Autodesk Inventor part; units mm, degrees
ref_plane "YZ Plane" through (0, 0, 0) normal (1, 0, 0) x (0, 1, 0)
ref_plane "XZ Plane" through (0, 0, 0) normal (0, 1, 0) x (-1, 0, 0)
ref_plane "XY Plane" through (0, 0, 0) normal (0, 0, 1) x (1, 0, 0)
sketch "Sketch1" plane through (0, 0, 0) normal (0, 1, 0) x (-1, 0, 0)
  line L0 (-13.25, -16.375) -> (13.25, -16.375)
  line L1 (13.25, -16.375) -> (13.25, 16.375)
  line L2 (13.25, 16.375) -> (-13.25, 16.375)
  line L3 (-13.25, 16.375) -> (-13.25, -16.375)
  line L4 (-13.25, -16.375) -> (13.25, 16.375) construction
  line L5 (13.25, -16.375) -> (-13.25, 16.375) construction
  point P0 (0, 0)
  dimension "d0" = 26.5
  dimension "d1" = 32.75
extrude "Extrusion1" add sketch "Sketch1" along normal blind 3.5 and the other way blind 11.5
shell "Shell1" thickness 1 removed faces 1 at (4.4167, -11.5, 5.4583)
sketch "Sketch2" plane through (0, 3.5, 0) normal (0, 1, 0) x (1, 0, 0)
  line L0 (13.25, 16.375) -> (-13.25, 16.375)
  line L1 (-13.25, 16.375) -> (-13.25, -16.375)
  line L2 (-13.25, -16.375) -> (13.25, -16.375)
  line L3 (13.25, -16.375) -> (13.25, 16.375)
  point P0 (0, 0)
extrude "Extrusion2" add sketch "Sketch2" along normal blind 1
sketch "Sketch3" plane through (-12.25, 2.5, -15.375) normal (0, -1, 0) x (1, 0, 0)
  line L0 (24.5, 0) -> (0, 0)
  line L1 (24.5, 30.75) -> (24.5, 0)
  line L2 (0, 30.75) -> (24.5, 30.75)
  line L3 (0, 0) -> (0, 30.75)
  line L4 (0.5, 3.625) -> (24, 3.625)
  line L5 (24, 3.625) -> (24, 27.125)
  line L6 (24, 27.125) -> (0.5, 27.125)
  line L7 (0.5, 27.125) -> (0.5, 3.625)
  circle A0 centre (12.25, 15.375) radius 11.75
  dimension "d9" = 0.5
  dimension "d10" = 0.5
  dimension "d11" = 3.625
  dimension "d12" = 3.625
  dimension "d13" = 23.5
  dimension "d14" = 23.5
extrude "Extrusion3" cut sketch "Sketch3" against normal blind 1 contours L7 A0 L4 | A0 L5 L4 | A0 | L7 L6 A0 | A0 L6 L5
extrude "Extrusion4" cut sketch "Sketch3" against normal blind 2 contours A0
sketch "Sketch4" plane through (-12.25, -11.5, -15.375) normal (0, 0, 1) x (1, 0, 0)
  line L0 (24.5, 0) -> (0, 0)
  line L1 (8.75, 6.5) -> (15.75, 6.5)
  line L2 (15.75, 6.5) -> (15.75, 0)
  line L3 (15.75, 0) -> (8.75, 0)
  line L4 (8.75, 0) -> (8.75, 6.5)
  line L5 (8.75, 6.5) -> (15.75, 0) construction
  line L6 (15.75, 6.5) -> (8.75, 0) construction
  circle A0 centre (12.25, 3.25) radius 3.5
  line L7 (15.75, 3.25) -> (15.75, 3.25)
  line L8 (8.75, 3.25) -> (8.75, 3.25)
  point P0 (12.25, 11.5)
  point P1 (12.25, 3.25)
  point P2 (12.25, 0)
  point P3 (12.25, 0)
  point P4 (10.951, 0)
  point P5 (13.549, 0)
  point P6 (15.75, 0)
  point P7 (15.75, 3.25)
  point P8 (8.75, 3.25)
  point P9 (8.75, 0)
  dimension "d19" = 7
  dimension "d20" = 6.5
  dimension "d21" = 7
  dimension "d22" = 3.25
  dimension "d23" = 3.25
extrude "Extrusion5" cut sketch "Sketch4" against normal blind 2 contours L0 A0 L2 | A0 L0 | L0 A0 L1 | L0 L4 A0 | L1 A0
sketch "Sketch5" plane through (-13.25, -11.5, -16.375) normal (-1, 0, 0) x (0, 0, 1)
  line L0 (0, 16) -> (32.75, 16)
  line L1 (30, 11) -> (3.2984, 11)
  line L2 (7, 11) -> (7, 3)
  line L3 (1, 0) -> (1, 14)
  line L4 (7, 4) -> (14, 4)
  line L5 (14, 4) -> (14, 11)
  line L6 (15.5, 11) -> (22.5, 11)
  line L7 (22.5, 11) -> (22.5, 4)
  line L8 (22.5, 4) -> (15.5, 4)
  line L9 (15.5, 4) -> (15.5, 11)
  point P0 (16.375, 11.5)
  dimension "d26" = 5
  dimension "d27" = 6
  dimension "d28" = 7
  dimension "d29" = 7
  dimension "d30" = 7
  dimension "d31" = 7
  dimension "d32" = 1.5
extrude "Extrusion6" cut sketch "Sketch5" against normal blind 2
sketch "Sketch6" plane through (0, -11.5, 0) normal (0, -1, 0) x (1, 0, 0)
  line L0 (3.5, -16.375) -> (13.25, -16.375)
  line L1 (13.25, -16.375) -> (13.25, 16.375)
  line L2 (13.25, 16.375) -> (-13.25, 16.375)
  line L3 (-13.25, 16.375) -> (-13.25, -16.375)
  line L4 (-13.25, -16.375) -> (-3.5, -16.375)
  line L5 (13.25, 16.375) -> (-13.25, 16.375)
  line L6 (-13.25, 16.375) -> (-13.25, -16.375)
  line L7 (-13.25, -16.375) -> (13.25, -16.375)
  line L8 (13.25, -16.375) -> (13.25, 16.375)
  point P0 (0, 0)
extrude "Extrusion7" add sketch "Sketch6" along normal blind 1
properties part number "carcasaXeotype_COLOR"
Part model, mm, in its own coordinate system. A direction names the side the tool comes from. Give positions to 0.01 mm unless a question says otherwise; leave off trailing zeros. Write each loop counter-clockwise with the first axis right and the second up, starting at its lowest first coordinate (ties: lowest second). Pieces come first, ordered by that corner, then holes.
1) Cut at B-B on x = -3. Write the cut outline in (y, z) (3 decimals), then the cut area to 3 significant figures.
Resolved:
outline: (-12.5, -16.375) - (-11.5, -16.375) - (-11.5, 15.375) - (2.5, 15.375) - (2.5, 11.75) - (3.5, 11.75) - (3.5, 11.361) - (4.5, 11.361) - (4.5, 16.375) - (-12.5, 16.375) - close; (-6.447, -16.375) - (4.5, -16.375) - (4.5, -11.361) - (3.5, -11.361) - (3.5, -11.75) - (2.5, -11.75) - (2.5, -15.375) - (-6.447, -15.375) - close
area: 75.0 mm2
2) Two-plate mould, pull along Z, no slides. Class faces 4 (the face through (-3.5, -10, -16)), 5 (the face through (0, -4, 16.375)), 6 (the face through (0, 3, -11.75)): released by +Z, released by -Z, zero draft, split by the parting line, or undercut.
Resolved:
face 4: zero draft
face 5: released by +Z
face 6: undercut
3) Cut at C-C on z = -10. Write the cut outline in (x, y).
Resolved:
outline: (-13.25, -12.5) - (13.25, -12.5) - (13.25, 4.5) - (6.17, 4.5) - (6.17, 3.5) - (11.75, 3.5) - (11.75, 2.5) - (12.25, 2.5) - (12.25, -11.5) - (-12.25, -11.5) - (-12.25, 2.5) - (-11.75, 2.5) - (-11.75, 3.5) - (-6.17, 3.5) - (-6.17, 4.5) - (-13.25, 4.5) - close
4) Cut at A-A on y = -1.75. Write the cut outline in (x, z) (3 decimals), then the cut area to 4 significant figures.
Resolved:
outline: (-13.25, -16.375) - (13.25, -16.375) - (13.25, 16.375) - (-13.25, 16.375) - (-13.25, 6.125) - (-12.25, 6.125) - (-12.25, 15.375) - (12.25, 15.375) - (12.25, -15.375) - (-12.25, -15.375) - (-12.25, -9.375) - (-13.25, -9.375) - close; (-13.25, -2.375) - (-12.25, -2.375) - (-12.25, -0.875) - (-13.25, -0.875) - close
area: 100.5 mm2
5) Cut at D-D on y = -9.75. Write the cut outline in (x, z) (3 decimals), then the cut area to 4 significant figures.
Resolved:
outline: (-13.25, -16.375) - (-3.5, -16.375) - (-3.5, -15.375) - (-12.25, -15.375) - (-12.25, 15.375) - (12.25, 15.375) - (12.25, -15.375) - (3.5, -15.375) - (3.5, -16.375) - (13.25, -16.375) - (13.25, 16.375) - (-13.25, 16.375) - close
area: 107.5 mm2
6) Probe L1, parallel to X at y = 4.25, z = 0; L2, parallel to X at y = -3.75, z = -14; L3, parallel to Z at x = -0.25, y = -0.25 (3 decimals). List the from-to ranges inside material, lowest first.
Resolved:
L1: x = -13.25 to -11.75, 11.75 to 13.25
L2: x = -13.25 to -12.25, 12.25 to 13.25
L3: z = -16.375 to -15.375, 15.375 to 16.375
7) Which spindle directions (+Z, -Z, +X, -X, +Y, -Y) get a long thin tool onto all of the face, cutting with end or side? Do faces 1 (the face through (3.5, -10, -16)), 2 (the face through (12, 2.5, -1)), 3 (the face through (-13, -4, -0.875)). Say none if no direction does.
Resolved:
face 1: -Z
face 2: none
face 3: -X
